Model file for the job. Use its own axes, mm. A direction names the side the tool comes from. Give positions to 0.01 mm unless a question says otherwise; leave off trailing zeros. Loops run counter-clockwise (first coordinate to the right, second up) from the corner with the lowest first, then second, coordinate; pieces in that order, holes last. Notation, with made-up numbers: M -19.75,-14.75 L 26.25,-14.75 A12 ccw 26.25,2.25 Z; hole C 13,67 d7. An arc over 180 degrees is marked long. Use CSV: the item, a comma, the result in double quotes. Start each with the question number.
(1) Slice it at A-A on y = -35.56. List the corners of the cut face in (x, z) (1 decimal), and give its area (3 significant figures).
(2) Flat gauge pins, fed straight in: P1, Ø1.8, axis at y = -16.51, z = 2.38, coming from the -X side; P2, Ø2.5, axis at y = -16.51, z = 2.38, coming from the -X side. Where does each tip first touch, or does it go through?
(3) Slice it at C-C on x = -8.5. List the corners of the cut face in (y, z).
(4) Wall check: line 1 along Y through (x, z) = (1, 1.7); line 2 along Y through (x, z) = (10, 3.3); line 3 along X through (y, z) = (32.5, 4.3) (1 decimal). Give the ranges that are in metal, low to high. Write a range as from..to.
(5) Tool access for faces 1 (the face through (0, 46.99, 2)), 2 (the face through (11.873, -18.103, 2.027)), 3 (the face through (-11.87, 36.68, 2.53)): list every direction of +Z, -Z, +X, -X, +Y, -Y with a clear straight run to the whole face (end or side of a thin tool).
(6) Two-plate mould, pull along X, no slides. Class faces 4 (the face through (8.53, 6.02, 2.35)), 5 (the face through (-14.288, -1, 2)), 6 (the face through (11.873, -34.184, 3.259)), 7 (the face through (14.288, -1, 2)): pulls with the +X half, pulls with the -X half, needs draft (parallel to the pull), parting line crosses it, or undercut.
(7) Slice it at B-B on x = 5.25. List the corners of the cut face in (y, z).
```python
from build123d import *

# Parameters (mm, degrees)
SKETCH1_W                 = 28.575
SKETCH1_H                 = 114.3
BOSS_EXTRUDE1_DEPTH       = 4.7625
SKETCH2_W                 = 19.05
SKETCH2_H                 = 41.91
CUT_EXTRUDE1_DEPTH        = 60.101070739
FILLET1_R                 = 3.302
F_4_CLEARANCE_HOLE1_D     = 3.2639
F_4_CLEARANCE_HOLE1_DEPTH = 4.7625
F_4_40_TAPPED_HOLE1_D     = 2.2606


with BuildPart() as part:
    # Sketch1 → Boss-Extrude1 (new body)
    with BuildSketch(Plane.XY):
        Rectangle(SKETCH1_W, SKETCH1_H)
    extrude(amount=BOSS_EXTRUDE1_DEPTH)

    # Sketch2 → Cut-Extrude1 (cut, through all)
    with BuildSketch(Plane.XY.offset(4.7625)):
        with Locations((0, 26.035)):
            Rectangle(SKETCH2_W, SKETCH2_H)
        with Locations((0, -26.035)):
            Rectangle(SKETCH2_W, SKETCH2_H)
    extrude(amount=-CUT_EXTRUDE1_DEPTH, mode=Mode.SUBTRACT)

    # Fillet1
    fillet1_edges = [part.edges().sort_by_distance(p)[0] for p in [
        (9.525, 46.99, 2.38125),
        (9.525, 5.08, 2.38125),
        (-9.525, 5.08, 2.38125),
        (-9.525, 46.99, 2.38125),
        (-9.525, -46.99, 2.38125),
        (-9.525, -5.08, 2.38125),
        (9.525, -5.08, 2.38125),
        (9.525, -46.99, 2.38125),
    ]]
    fillet(fillet1_edges, radius=FILLET1_R)

    # #4 Clearance Hole1
    with Locations(Plane(origin=(14.2875, 0, 0), x_dir=(0, 0, -1), z_dir=(1, 0, 0))):
        with Locations((-2.38125, 35.56), (-2.38125, 16.51), (-2.38125, -16.51), (-2.38125, -35.56)):
            Hole(F_4_CLEARANCE_HOLE1_D / 2, depth=F_4_CLEARANCE_HOLE1_DEPTH)

    # #4-40 Tapped Hole1 (through all)
    with Locations(Plane.ZY.offset(14.2875)):
        with Locations((2.38125, 16.51), (2.38125, 35.56), (2.38125, -16.51), (2.38125, -35.56)):
            Hole(F_4_40_TAPPED_HOLE1_D / 2)


solid = part.part
```
Reply:
1,outline,"M -14.3,0 L -9.5,0 L -9.5,1.3 L -14.3,1.3 Z; M -14.3,3.5 L -9.5,3.5 L -9.5,4.8 L -14.3,4.8 Z; M 9.5,0 L 14.3,0 L 14.3,0.7 L 9.5,0.7 Z; M 9.5,4 L 14.3,4 L 14.3,4.8 L 9.5,4.8 Z"
1,area,"19.1 mm^2"
2,P1,"passes through"
2,P2,"stops at x = -14.29"
3,outline,"M -57.15,0 L -46.08,0 L -46.08,4.76 L -57.15,4.76 Z; M -5.99,0 L 5.99,0 L 5.99,4.76 L -5.99,4.76 Z; M 46.08,0 L 57.15,0 L 57.15,4.76 L 46.08,4.76 Z"
4,line 1,"y = -57.15..-46.99, -5.08..5.08, 46.99..57.15"
4,line 2,"y = -57.15..-36.91, -34.21..-17.86, -15.16..15.16, 17.86..34.21, 36.91..57.15"
4,line 3,"x = -14.3..-9.5, 9.5..14.3"
5,face 1,"+Z, -Z"
5,face 2,"+X"
5,face 3,"+X, -X"
6,face 4,"undercut"
6,face 5,"pulls with the -X half"
6,face 6,"needs draft"
6,face 7,"pulls with the +X half"
7,outline,"M -57.15,0 L -46.99,0 L -46.99,4.76 L -57.15,4.76 Z; M -5.08,0 L 5.08,0 L 5.08,4.76 L -5.08,4.76 Z; M 46.99,0 L 57.15,0 L 57.15,4.76 L 46.99,4.76 Z"
